from build123d import *

# Parameters (mm, degrees)
F0_W           = 46.3467240334
F0_H           = 115.6897172332
F1_DEPTH       = 25
F2_R           = 12
F4_DEPTH       = 40
F4_DEPTH_BACK  = 40
F6_R           = 17.7712313218
F7_DEPTH       = 10
F8_R           = 23.1733620167
F9_DEPTH       = 25
F11_R          = 21.9307918762
F12_DEPTH      = 25
F14_DEPTH      = 15
F14_DEPTH_BACK = 15
F15_T          = 2.5
F16_R          = 15.8642477534
F17_DEPTH      = 25
F18_DEPTH      = 5
F19_DEPTH      = 25
F20_T1_DEPTH   = 101.1275982577
F20_T3_DEPTH   = 92.184276345
F20_T5_DEPTH   = 22.3467240334
F20_T8_ANGLE   = 90
F20_T12_DEPTH  = 92.184276345
F20_T17_DEPTH  = 92.184276345
F20_T22_DEPTH  = 92.184276345
F20_T27_DEPTH  = 101.1275982577
F20_T30_ANGLE  = 90
F21_W          = 30.3467240334
F21_H          = 11.4395302832
F22_DEPTH      = 10
F23_SIZE       = 5


# Not quite as in the source:
# - a fillet or chamfer that OpenCascade refuses, or shapes differently, is made with other operations: its cross-section is extruded or revolved along the edge and cut away or added
# - a shell that OpenCascade refuses in one call is made with other operations: the cavity is built on its own and cut out


with BuildPart() as f1:
    # F0 (on Top) → F1 (new body)
    with BuildSketch(Plane.XY):
        with Locations((7.814258337, 1.8636099994)):
            Rectangle(F0_W, F0_H)
    extrude(amount=F1_DEPTH)

    # F2
    f2_edges = [f1.edges().sort_by_distance(p)[0] for p in [
        (30.98762, -55.981249, 12.5),
        (-15.359104, -55.981249, 12.5),
    ]]
    fillet(f2_edges, radius=F2_R)

    # F3 (on Right) → F4 (cut, two sides)
    with BuildSketch(Plane.YZ) as f4_sk:
        Polygon((0, 31.970962882), (68.2880878448, 11.4047080278), (67.6364898682, 28.4685865045), align=None)
    extrude(amount=F4_DEPTH, mode=Mode.SUBTRACT)
    extrude(f4_sk.sketch, amount=-F4_DEPTH_BACK, mode=Mode.SUBTRACT)


with BuildPart() as f1_1:
    # F5: moved
    add(f1.part.moved(Location((-7.1676671505, 0, 0))))

    # F6 (on face) → F7 (cut)
    with BuildSketch(Plane.XY.offset(25)):
        with Locations((0, -12.5934332609)):
            Circle(F6_R)
    extrude(amount=-F7_DEPTH, mode=Mode.SUBTRACT)

    # F15: shell of thickness 2.5, made by hand


with BuildPart() as f9:
    # F8 (on face) → F9 (new body)
    with BuildSketch(Plane(origin=(0, 59.708468616, 0), x_dir=(-1, 0, 0), z_dir=(0, 1, 0))):
        with Locations((-0.6465911865, 33.9257717133)):
            Circle(F8_R)
    extrude(amount=-F9_DEPTH)


with BuildPart() as f9_1:
    # F10: moved
    add(f9.part.moved(Location((0, 0, 10.7776373625))))

    # F11 (on face) → F12 (cut)
    with BuildSketch(Plane(origin=(0, 59.708468616, 0), x_dir=(-1, 0, 0), z_dir=(0, 1, 0))):
        with Locations((-0.6465911865, 44.7034090757)):
            Circle(F11_R)
    extrude(amount=-F12_DEPTH, mode=Mode.SUBTRACT)


with BuildPart() as f14:
    # F13 (on Right) → F14 (new body, two sides)
    with BuildSketch(Plane.YZ) as f14_sk:
        Polygon((59.624966234, 14.1331925988), (59.624966234, 21.5853508562), (34.9215567112, 21.3780961931), align=None)
    extrude(amount=F14_DEPTH)
    extrude(f14_sk.sketch, amount=-F14_DEPTH_BACK)


with BuildPart() as f15_core1:
    # F15_t2: copy of F1
    add(f1_1.part)

    # the walls: a layer under each face that stays
    f15_faces = [f15_core1.faces().sort_by_distance(p)[0] for p in [
        (-22.5267708302, 7.8636099994, 12.5),
        (-19.0120522044, -52.4665299914, 12.5),
        (-14.8023168246, -42.7933155742, 25),
        (0.6465911865, 41.4274091283, 19.4943116685),
        (0.6465911865, 59.708468616, 6.9943116685),
        (0.6465911865, -55.9812486172, 12.5),
        (23.8199532032, 7.8636099994, 12.5),
        (20.3052345774, -52.4665299914, 12.5),
        (-17.7712313218, -12.5934332609, 20),
        (0, -12.5934332609, 15),
    ]]
    thicken(f15_faces, amount=-F15_T, mode=Mode.SUBTRACT)

    # F15_s3 → F15_t4 (revolve, cut)
    with BuildSketch(Plane.XZ.offset(12.5934332609)):
        Polygon((17.7462313218, 15.025), (20.2712313218, 15), (20.2712313218, 12.5), (17.7712313218, 12.5), align=None)
    revolve(axis=Axis((0, -12.5934332609, 15), (0, 0, 1)), mode=Mode.SUBTRACT)


with BuildPart() as f1_2:
    add(f1_1.part)

    # what is left inside the walls is the cavity
    f15_cavity = [f15_core1.part.solids().sort_by_distance(p)[0] for p in [
        (0.646591, -16.584676, 0.025),
    ]]
    add(f15_cavity, mode=Mode.SUBTRACT)

    # F16 (on face) → F17 (cut)
    with BuildSketch(Plane.XY.offset(15)):
        with Locations((0, -12.5934332609)):
            Circle(F16_R)
    extrude(amount=-F17_DEPTH, mode=Mode.SUBTRACT)

    # F18 (add): a face of the model
    f18_faces = [f14.part.faces().sort_by_distance(p)[0] for p in [
        (0, 47.2732614726, 21.4817235246),
    ]]

    add(f9_1.part)  # F18 merges F9

    add(f14.part)  # F18 merges F14
    extrude(f18_faces, amount=F18_DEPTH)

    # F11 (on face) → F19 (cut)
    with BuildSketch(Plane(origin=(0, 59.708468616, 0), x_dir=(-1, 0, 0), z_dir=(0, 1, 0))):
        with Locations((-0.6465911865, 44.7034090757)):
            Circle(F11_R)
    extrude(amount=-F19_DEPTH, mode=Mode.SUBTRACT)

    # F20: fillet of radius 8 on 7 edges, made by hand

    # F20_s2 → F20_t1 (cut)
    with BuildSketch(Plane.XZ.offset(-57.1463496406)):
        with BuildLine():
            ThreePointArc((15.8199532032, 25), (21.4768074527, 22.6568542495), (23.8199532032, 17))
            Line((23.8199532032, 17), (23.8199532032, 25))
            Line((23.8199532032, 25), (15.8199532032, 25))
        make_face()
    extrude(amount=F20_T1_DEPTH, mode=Mode.SUBTRACT)

    # F20_s4 → F20_t3 (cut)
    with BuildSketch(Plane(origin=(0, -18.2371947161, 5.4924776223), x_dir=(1, 0, 0), z_dir=(0, 0.9575176611, -0.2883746326))):
        with BuildLine():
            ThreePointArc((15.8199532032, -30.6127616009), (21.4768074527, -28.2696158504), (23.8199532032, -22.6127616009))
            Line((23.8199532032, -22.6127616009), (23.8199532032, -30.6127616009))
            Line((23.8199532032, -30.6127616009), (15.8199532032, -30.6127616009))
        make_face()
    extrude(amount=F20_T3_DEPTH, mode=Mode.SUBTRACT)

    # F20_s6 → F20_t5 (cut)
    with BuildSketch(Plane.YZ.offset(-10.5267708302)):
        with BuildLine():
            ThreePointArc((-47.9812486172, 25), (-53.6381028667, 22.6568542495), (-55.9812486172, 17))
            Line((-55.9812486172, 17), (-55.9812486172, 25))
            Line((-55.9812486172, 25), (-47.9812486172, 25))
        make_face()
    extrude(amount=F20_T5_DEPTH, mode=Mode.SUBTRACT)

    # F20_s7 → F20_t8 (revolve, cut)
    with BuildSketch(Plane.YZ.offset(11.8199532032)):
        with BuildLine():
            ThreePointArc((-47.9812486172, 25), (-53.6381028667, 22.6568542495), (-55.9812486172, 17))
            Line((-55.9812486172, 17), (-55.9812486172, 25))
            Line((-55.9812486172, 25), (-47.9812486172, 25))
        make_face()
    revolve(axis=Axis((11.8199532032, -43.9812486172, 25), (0, 0, 1)), revolution_arc=F20_T8_ANGLE, mode=Mode.SUBTRACT)


with BuildPart() as f20_tool10:
    # F20_s11 → F20_t12 (new body)
    with BuildSketch(Plane(origin=(0, 70.0308779571, -21.0911292025), x_dir=(1, 0, 0), z_dir=(0, -0.9575176611, 0.2883746326))):
        with BuildLine():
            ThreePointArc((-14.5267708302, 30.6127616009), (-20.1836250796, 28.2696158504), (-22.5267708302, 22.6127616009))
            Line((-22.5267708302, 22.6127616009), (-22.5267708302, 30.6127616009))
            Line((-22.5267708302, 30.6127616009), (-14.5267708302, 30.6127616009))
        make_face()
    extrude(amount=F20_T12_DEPTH)

    split(bisect_by=Plane(origin=(0, 8.5388595544, 29.1154936273), x_dir=(1, 0, 0), z_dir=(0, -0.281422426, -0.9595839818)), keep=Keep.TOP)


with BuildPart() as f1_3:
    add(f1_2.part)

    # F20_t9: cut F20_tool10
    add(f20_tool10.part, mode=Mode.SUBTRACT)


with BuildPart() as f20_tool15:
    # F20_s16 → F20_t17 (new body)
    with BuildSketch(Plane(origin=(0, 70.0308779571, -21.0911292025), x_dir=(1, 0, 0), z_dir=(0, -0.9575176611, 0.2883746326))):
        with BuildLine():
            ThreePointArc((-14.5267708302, 30.6127616009), (-20.1836250796, 28.2696158504), (-22.5267708302, 22.6127616009))
            Line((-22.5267708302, 22.6127616009), (-22.5267708302, 30.6127616009))
            Line((-22.5267708302, 30.6127616009), (-14.5267708302, 30.6127616009))
        make_face()
    extrude(amount=F20_T17_DEPTH)

    split(bisect_by=Plane.YZ.offset(-15), keep=Keep.BOTTOM)


with BuildPart() as f1_4:
    add(f1_3.part)

    # F20_t14: cut F20_tool15
    add(f20_tool15.part, mode=Mode.SUBTRACT)


with BuildPart() as f20_tool20:
    # F20_s21 → F20_t22 (new body)
    with BuildSketch(Plane(origin=(0, 70.0308779571, -21.0911292025), x_dir=(1, 0, 0), z_dir=(0, -0.9575176611, 0.2883746326))):
        with BuildLine():
            ThreePointArc((-14.5267708302, 30.6127616009), (-20.1836250796, 28.2696158504), (-22.5267708302, 22.6127616009))
            Line((-22.5267708302, 22.6127616009), (-22.5267708302, 30.6127616009))
            Line((-22.5267708302, 30.6127616009), (-14.5267708302, 30.6127616009))
        make_face()
    extrude(amount=F20_T22_DEPTH)

    split(bisect_by=Plane(origin=(0, 35.0984424425, 0.2944660678), x_dir=(1, 0, 0), z_dir=(0, -0.9999648082, -0.0083894237)), keep=Keep.TOP)


with BuildPart() as f1_5:
    add(f1_4.part)

    # F20_t19: cut F20_tool20
    add(f20_tool20.part, mode=Mode.SUBTRACT)


with BuildPart() as f20_tool25:
    # F20_s26 → F20_t27 (new body)
    with BuildSketch(Plane.XZ.offset(-57.1463496406)):
        with BuildLine():
            ThreePointArc((-22.5267708302, 17), (-20.1836250796, 22.6568542495), (-14.5267708302, 25))
            Line((-14.5267708302, 25), (-22.5267708302, 25))
            Line((-22.5267708302, 25), (-22.5267708302, 17))
        make_face()
    extrude(amount=F20_T27_DEPTH)

    split(bisect_by=Plane(origin=(0, 8.8279438803, 29.312259887), x_dir=(1, 0, 0), z_dir=(0, -0.2883746326, -0.9575176611)), keep=Keep.TOP)


with BuildPart() as f1_6:
    add(f1_5.part)

    # F20_t24: cut F20_tool25
    add(f20_tool25.part, mode=Mode.SUBTRACT)

    # F20_s29 → F20_t30 (revolve, cut)
    with BuildSketch(Plane.XZ.offset(43.9812486172)):
        with BuildLine():
            ThreePointArc((-14.5267708302, 25), (-20.1836250796, 22.6568542495), (-22.5267708302, 17))
            Line((-22.5267708302, 17), (-22.5267708302, 25))
            Line((-22.5267708302, 25), (-14.5267708302, 25))
        make_face()
    revolve(axis=Axis((-10.5267708302, -43.9812486172, 25), (0, 0, 1)), revolution_arc=F20_T30_ANGLE, mode=Mode.SUBTRACT)

    # F21 (on face) → F22 (join)
    with BuildSketch(Plane.XY.offset(25)):
        with Locations((0.6465911865, -38.2614834756)):
            Rectangle(F21_W, F21_H)
    extrude(amount=F22_DEPTH)

    # F23
    f23_edges = [f1_6.edges().sort_by_distance(p)[0] for p in [
        (15.819953, -38.261483, 35),
        (-14.526771, -38.261483, 35),
        (0.646591, -43.981249, 35),
    ]]
    chamfer(f23_edges, length=F23_SIZE)


solid = f1_6.part
Check sheet for the modelled part. Datum: model origin and axes. Units: mm. A direction names the side the tool comes from. Round coordinates to 2 decimals unless told otherwise and drop trailing zeros. Order: outer loops, then holes, each group sorted by start corner. A loop starts at its lowest first (then second) coordinate and runs counter-clockwise, first axis right, second up.
Q1. Depth check by flat-ended pin: P1, Ø7, axis at x = 1.5, y = -35, coming from the +Z side; P2, Ø3, axis at x = 13.5, y = -27, coming from the -Z side; P3, Ø5, axis at x = 5, z = 28, coming from the +Y side. Enter the tip coordinate at first touch or a pass-through.
Filled sheet:
P1: stops at z = 35
P2: stops at z = 12.5
P3: stops at y = -32.54
Q2. Cross-section at A-A, the plane z = 60. Enter the section's corners in (x, y).
Filled sheet:
outline: (-16.76, 34.71) - (-15.07, 34.71) - (-15.07, 59.71) - (-16.76, 59.71) - close; (16.36, 34.71) - (18.05, 34.71) - (18.05, 59.71) - (16.36, 59.71) - close
Q3. Draft check along Z on faces 6 (the face through (21.414, 41.651, 17.044)), 7 (the face through (0.49, -53.576, 22.719)), 8 (the face through (21.32, 6, 11)). Enter one of: pulls with the +Z half, pulls with the -Z half, needs draft (parallel to the pull), parting line crosses it, or undercut.
Filled sheet:
face 6: undercut
face 7: pulls with the +Z half
face 8: needs draft
Q4. Scan lines: L1, parallel to Z at x = 17, y = 40; L2, parallel to Z at x = -8, y = -30; L3, parallel to Y at x = 4.5, z = 7. Record each from-to range of solid material in increasing order.
Filled sheet:
L1: z = 17.31 to 19.83, 28.28 to 30.09, 59.32 to 61.12
L2: z = 12.5 to 25
L3: y = -55.98 to -53.48, 57.21 to 59.71
Q5. Cross-section at B-B, the plane x = -4.5. Give the number of separate pieces and of enclosed holes in the cut face, plus the area to 3 significant figures.
Filled sheet:
separate pieces: 3
enclosed holes: 0
area: 613 mm2
Q6. Cross-section at C-C, the plane z = 50.5. Enter the section's corners in (x, y).
Filled sheet:
outline: (-21.79, 34.71) - (-20.5, 34.71) - (-20.5, 59.71) - (-21.79, 59.71) - close; (21.8, 34.71) - (23.08, 34.71) - (23.08, 59.71) - (21.8, 59.71) - close
Q7. Set-up check for faces 1 (the face through (-7, 2, 15)), 2 (the face through (0, -43.981, 27)), 3 (the face through (10, -32, 22.5)), 4 (the face through (-15, 50, 22)), 5 (the face through (15.82, -38, 27)): record each of +Z, -Z, +X, -X, +Y, -Y from which the full face is reachable in a straight line by a thin tool's end or side.
Filled sheet:
face 1: +Z
face 2: +Z, +X, -X, -Y
face 3: -Z
face 4: -X, +Y
face 5: +Z, +X, -Y
